Check sheet for the modelled part. Datum: model origin and axes. Units: mm. A direction names the side the tool comes from. Round coordinates to 2 decimals unless told otherwise and drop trailing zeros. Write each loop counter-clockwise with the first axis right and the second up, starting at its lowest first coordinate (ties: lowest second). Pieces come first, ordered by that corner, then holes. Notation, with made-up numbers: (-16.75, 44.25) - (6.25, 44.25) arc R34 cw to (6.25, 82.25) - close; hole circle Ø10 at (46.5, 32). An arc over 180 degrees is marked (long way). Answer as a JSON object with one key per item and string values. Group by question number.
Item 1: Sectioned sample at D-D on z = 22.75. Record the boundary of the cut face in (x, y) (3 decimals).
Item 2: Sectioned sample at A-A on z = 12.7. Count the separate pieces of the cut face and the enclosed holes in it, plus the area to 3 significant figures.
Item 3: Sectioned sample at C-C on x = -46.5. Record the boundary of the cut face in (y, z).
Item 4: Release check for a two-part mould opening along X. For faces 3 (the flat face through (-44, 6.35, 13)), 4 (the flat face through (-63, 57.15, 16)), 5 (the flat face through (0, 3, 13)), 6 (the flat face through (-111.125, 3, 13)) record: pulls with the +X half, pulls with the -X half, needs draft (parallel to the pull), parting line crosses it, or undercut.
Item 5: Set-up check for faces 1 (the cylindrical face through (-28.01, 3.22, 14.07)), 2 (the cylindrical face through (-59.437, 31.394, 11.708)): record each of +Z, -Z, +X, -X, +Y, -Y from which the full face is reachable in a straight line by a thin tool's end or side.
Item 6: Sectioned sample at B-B on y = 43. Record the boundary of the cut face in (x, z) (1 decimal).
Item 7: Gauge pin test, flat ends, axial feed: P1, Ø1.5, axis at y = 47.5, z = 16, coming from the -X side; P2, Ø1, axis at x = -63, y = 16, coming from the -Z side; P3, Ø1, axis at x = -53, y = 42.5, coming from the -Z side; P4, Ø6.5, axis at x = -30.16, z = 12.7, coming from the +Y side. Record the tip position at first contact, or that the pin passes through.
Item 8: Thickness scan on line 1 (X direction, y = 21, z = 12.7) (1 decimal); line 2 (Z direction, x = -44, y = 54); line 3 (X direction, y = 30, z = 11.75). Record the ranges inside material, lowest first.
```python
from build123d import *

# Parameters (mm, degrees)
SKETCH1_W           = 111.125
SKETCH1_H           = 25.4
BOSS_EXTRUDE1_DEPTH = 6.35
SKETCH2_R           = 7.62
SKETCH2_R_2         = 4.7625
BOSS_EXTRUDE2_DEPTH = 50.8
SKETCH2_9_R         = 2.5527
CUT_EXTRUDE1_DEPTH  = 125.798099445


with BuildPart() as part:
    # Sketch1 → Boss-Extrude1 (new body)
    with BuildSketch(Plane(origin=(0, 0, 0), x_dir=(1, 0, 0), z_dir=(0, 1, 0))):
        with Locations((-55.5625, -12.7)):
            Rectangle(SKETCH1_W, SKETCH1_H)
    extrude(amount=BOSS_EXTRUDE1_DEPTH)

    # Sketch2 → Boss-Extrude2 (add)
    # profile 1 of 2: a face of its own
    with BuildSketch(Plane(origin=(0, 6.35, 0), x_dir=(1, 0, 0), z_dir=(0, 1, 0))):
        with Locations(Location((-44.1325, -12.7, 0), (0, 0, 270))):
            Circle(SKETCH2_R)
        with Locations(Location((-44.1325, -12.7, 0), (0, 0, 270))):
            Circle(SKETCH2_R_2, mode=Mode.SUBTRACT)
    # profile 2 of 2: a face of its own
    with BuildSketch(Plane(origin=(0, 6.35, 0), x_dir=(1, 0, 0), z_dir=(0, 1, 0))):
        with Locations(Location((-66.9925, -12.7, 0), (0, 0, 270))):
            Circle(SKETCH2_R)
        with Locations(Location((-66.9925, -12.7, 0), (0, 0, 270))):
            Circle(SKETCH2_R_2, mode=Mode.SUBTRACT)
    extrude(amount=BOSS_EXTRUDE2_DEPTH)

    # Sketch2_9 → Cut-Extrude1 (cut, through all)
    with BuildSketch(Plane(origin=(0, 6.35, 0), x_dir=(1, 0, 0), z_dir=(0, 1, 0))):
        with Locations(Location((-30.1625, -12.7, 0), (0, 0, 270))):
            Circle(SKETCH2_9_R)
        with Locations(Location((-80.9625, -12.7, 0), (0, 0, 270))):
            Circle(SKETCH2_9_R)
    extrude(amount=-CUT_EXTRUDE1_DEPTH, mode=Mode.SUBTRACT)


solid = part.part
```
Completed:
{
 "1": {"outline": "(-111.125, 0) - (0, 0) - (0, 6.35) - (-111.125, 6.35) - close"},
 "2": {"separate pieces": "3", "enclosed holes": "0", "area": "1,220 mm²"},
 "3": {"outline": "(0, 0) - (6.35, 0) - (6.35, 5.46) - (57.15, 5.46) - (57.15, 8.57) - (6.35, 8.57) - (6.35, 16.83) - (57.15, 16.83) - (57.15, 19.94) - (6.35, 19.94) - (6.35, 25.4) - (0, 25.4) - close"},
 "4": {"face 3": "undercut", "face 4": "needs draft", "face 5": "pulls with the +X half", "face 6": "pulls with the -X half"},
 "5": {"face 1": "+Y, -Y", "face 2": "+Y"},
 "6": {"outline": "circle Ø15.2 at (-67, 12.7); circle Ø15.2 at (-44.1, 12.7); hole circle Ø9.5 at (-67, 12.7); hole circle Ø9.5 at (-44.1, 12.7)"},
 "7": {"P1": "x = -74.17", "P2": "z = 5.93", "P3": "through", "P4": "y = 6.35"},
 "8": {"line 1": "-74.6 to -71.8, -62.2 to -59.4, -51.8 to -48.9, -39.4 to -36.5", "line 2": "5.08 to 7.94, 17.46 to 20.32", "line 3": "-74.55 to -71.66, -62.33 to -59.43, -51.69 to -48.8, -39.47 to -36.57"}
}
